Build history of the part. All positions in model axes, mm. A direction names the side the tool comes from. Round coordinates to 2 decimals unless told otherwise and drop trailing zeros. Loops run counter-clockwise (first coordinate to the right, second up) from the corner with the lowest first, then second, coordinate; pieces in that order, holes last. Notation, with made-up numbers: (-11.75, 16) -> (-0.75, 16) arc R23 cw to (-0.75, 35) -> close; hole circle Ø4 at (-16.75, -38). An arc over 180 degrees is marked (long way). Put each result on its own line as item: value. Start each with the question number.
Item 1: Drill centre lines: probe 1 along Y at (x, z) = (60, 2.4); probe 2 along Z at (x, y) = (103.5, 24.75); probe 3 along Y at (x, z) = (5, 3). Where is each one in solid material? Low to high. Write a range as [from, to].
Item 2: Cut at B-B, the plane x = 101. List the corners of the cut face in (y, z).
Item 3: Flat gauge pins, fed straight in: pin 1 Ø0.9 at (x, z) = (30, 2.5) entering from +Y; pin 2 Ø0.9 at (x, z) = (67, 2.5) entering from -Y; pin 3 Ø1.6 at (x, y) = (27.5, 0.5) entering from +Z. Where does each tip first touch, or does it go through?
Item 4: Tool access for faces 1 (the flat face through (53, 26, 1.5)), 2 (the flat face through (53, 1, 1.5)), 3 (the flat face through (53, 13, 0)): list every direction of +Z, -Z, +X, -X, +Y, -Y with a clear straight run to the whole face (end or side of a thin tool).
Item 5: Cut at A-A, the plane y = 17.75. List the corners of the cut face in (x, z), plus the area to 3 significant figures.
Item 6: Pull direction Y, two halves, no side cores. Call faces 4 (the cylindrical face through (102.34, 21.36, 1.65)), 5 (the flat face through (53, 24.5, 2)), 6 (the flat face through (53, 2, 2)), 7 (the flat face through (53, 13, 3.25)): +Y half, -Y half, draft (parallel to the pull), parting line (faces both ways), or undercut.
```python
from build123d import *

# Parameters (mm, degrees)
SKETCH_W     = 108
SKETCH_H     = 26.5
PAD_DEPTH    = 1.5
SKETCH001_W  = 108
SKETCH001_H  = 22.5
PAD001_DEPTH = 1.75
SKETCH002_R  = 2.5
POCKET_DEPTH = 3.251


with BuildPart() as part:
    # Sketch → Pad (new body)
    with BuildSketch(Plane.XY):
        with Locations((54, 13.25)):
            Rectangle(SKETCH_W, SKETCH_H)
    extrude(amount=PAD_DEPTH)

    # Sketch001 (on Face6 of Pad) → Pad001 (join)
    with BuildSketch(Plane.XY.offset(1.5)):
        with Locations((54, 13.25)):
            Rectangle(SKETCH001_W, SKETCH001_H)
    extrude(amount=PAD001_DEPTH)

    # Sketch002 (on Face12 of Pad001) → Pocket (cut, through all)
    with BuildSketch(Plane.XY.offset(3.25)):
        with Locations((101, 19.25)):
            Circle(SKETCH002_R)
        with Locations((7, 17.75)):
            Circle(SKETCH002_R)
    extrude(amount=-POCKET_DEPTH, mode=Mode.SUBTRACT)


solid = part.part
```
Reply:
1. probe 1: y = [2, 24.5]
1. probe 2: z = [0, 1.5]
1. probe 3: y = [2, 16.25], [19.25, 24.5]
2. outline: (0, 0) -> (16.75, 0) -> (16.75, 3.25) -> (2, 3.25) -> (2, 1.5) -> (0, 1.5) -> close; (21.75, 0) -> (26.5, 0) -> (26.5, 1.5) -> (24.5, 1.5) -> (24.5, 3.25) -> (21.75, 3.25) -> close
3. pin 1: stops at y = 24.5
3. pin 2: stops at y = 2
3. pin 3: stops at z = 1.5
4. face 1: +Z, +X, -X, +Y
4. face 2: +Z, +X, -X, -Y
4. face 3: -Z, +X, -X, +Y, -Y
5. outline: (0, 0) -> (4.5, 0) -> (4.5, 3.25) -> (0, 3.25) -> close; (9.5, 0) -> (99, 0) -> (99, 3.25) -> (9.5, 3.25) -> close; (103, 0) -> (108, 0) -> (108, 3.25) -> (103, 3.25) -> close
5. area: 322 mm^2
6. face 4: undercut
6. face 5: +Y half
6. face 6: -Y half
6. face 7: draft
